Read the model definition and answer for the solid it produces. Units are mm, in the model's axes. A direction names the side the tool comes from. Round coordinates to 2 decimals unless told otherwise and drop trailing zeros. Write each loop counter-clockwise with the first axis right and the second up, starting at its lowest first coordinate (ties: lowest second). Pieces come first, ordered by that corner, then holes. Notation, with made-up numbers: (9, -32) -> (21, -32) arc R31 cw to (21, -3) -> close; hole circle Ø5 at (12.5, 20). An arc over 180 degrees is marked (long way). Return JSON: item names as keys, results as strings.
Autodesk Inventor part; units mm, degrees
ref_plane "YZ Plane" through (0, 0, 0) normal (1, 0, 0) x (0, 1, 0)
ref_plane "XZ Plane" through (0, 0, 0) normal (0, 1, 0) x (-1, 0, 0)
ref_plane "XY Plane" through (0, 0, 0) normal (0, 0, 1) x (1, 0, 0)
sketch "Эскиз1" plane through (0, 0, 0) normal (0, 1, 0) x (-1, 0, 0)
  line L0 (0, 0) -> (-2.8, 0)
  line L1 (0, 0) -> (0, -6)
  line L2 (0, -6) -> (-1.3212, -6)
  line L3 (-1.45, -5.8712) -> (-1.45, -1.65)
  line L4 (-2.8, -0.3) -> (-1.45, -1.65)
  line L5 (-2.8, 0) -> (-2.8, -0.3)
  line L6 (-1.45, -5.8712) -> (-1.3212, -6)
revolve "Вращение1" add sketch "Эскиз1" angle 360 about axis through (0, 0, 0) along (0, 0, -1)
sketch "Эскиз2" plane through (0, 0, 0) normal (0, 0, 1) x (1, 0, 0)
  line L0 (-1.3212, -0.4705) -> (-1.3212, 0.4705)
  line L1 (1.3212, 0.4705) -> (1.3212, -0.4705)
  circle A0 centre (0, 0) radius 1.45
  line L2 (0.4865, -1.366) -> (-0.4865, -1.366)
  line L3 (-0.4865, 1.366) -> (0.4865, 1.366)
  line L4 (1.3212, -0.4705) -> (0.4865, -0.4705)
  line L5 (-0.4865, -0.4705) -> (-1.3212, -0.4705)
  line L6 (-0.4865, -1.366) -> (-0.4865, -0.4705)
  line L7 (-0.4865, 0.4705) -> (-0.4865, 1.366)
  line L8 (-1.3212, 0.4705) -> (-0.4865, 0.4705)
  line L9 (0.4865, 0.4705) -> (1.3212, 0.4705)
  line L10 (0.4865, 1.366) -> (0.4865, 0.4705)
  line L11 (0.4865, -0.4705) -> (0.4865, -1.366)
extrude "Выдавливание1" cut sketch "Эскиз2" against normal blind 1 contours L0 L8 L7 L3 L10 L9 L1 L4 L11 L2 L6 L5
thread "Резьба1"
properties part number "Винт М3х6 пот"
Item 1: Section C-C (x = 0) is taken. Give the vertices of the cut face in (y, z), then the cut area to 3 significant figures.
Worked answers:
{"outline": "(-2.8, -0.3) -> (-1.45, -1.65) -> (-1.45, -5.87) -> (-1.32, -6) -> (1.32, -6) -> (1.45, -5.87) -> (1.45, -1.65) -> (2.8, -0.3) -> (2.8, 0) -> (1.37, 0) -> (1.37, -1) -> (-1.37, -1) -> (-1.37, 0) -> (-2.8, 0) -> close", "area": "17.3 mm2"}
Item 2: Section D-D (z = -2.75) is taken. Give the vertices of the cut face in (x, y), then the cut area to 3 significant figures.
Worked answers:
{"outline": "circle Ø2.9 at (0, 0)", "area": "6.61 mm2"}
Item 3: Straight lines are drawn through the part: L1, parallel to X at y = -0.05, z = -0.25; L2, parallel to Y at x = 0.05, z = -1.7; L3, parallel to Z at x = -0.1, y = 2.1. For each, find the intervals that lie inside material, in ascending order. Write a range as [from, to].
Worked answers:
{"L1": "x = [-2.8, -1.32], [1.32, 2.8]", "L2": "y = [-1.45, 1.45]", "L3": "z = [-1, 0]"}
Item 4: A tool of negligible diameter and unlimited length cuts with its end or side. For faces 4 (the flat face through (-0.9, -0.47, -0.5)), 5 (the flat face through (1, 1, 0)), from which of +Z, -Z, +X, -X, +Y, -Y can it reach the whole face along a straight path? Write none if from no direction.
Worked answers:
{"face 4": "+Z", "face 5": "+Z, +X, -X, +Y, -Y"}
Item 5: Section A-A (z = -0.5) is taken. Give the vertices of the cut face in (x, y), then the cut area to 3 significant figures.
Worked answers:
{"outline": "circle Ø5.2 at (0, 0); hole (-1.32, -0.47) -> (-0.49, -0.47) -> (-0.49, -1.37) -> (0.49, -1.37) -> (0.49, -0.47) -> (1.32, -0.47) -> (1.32, 0.47) -> (0.49, 0.47) -> (0.49, 1.37) -> (-0.49, 1.37) -> (-0.49, 0.47) -> (-1.32, 0.47) -> close", "area": "17.0 mm2"}
Item 6: For a pull along X with two mould halves and no side action, classify faces 1 (the cylindrical face through (-1.45, 0.06, -3.73)), 2 (the flat face through (0, 0, -6)), 3 (the flat face through (0.486, 0.9, -0.5)) as released by +X, released by -X, zero draft, split by the parting line, or undercut.
Worked answers:
{"face 1": "split by the parting line", "face 2": "zero draft", "face 3": "undercut"}
Item 7: Section B-B (y = 0) is taken. Give the vertices of the cut face in (x, z).
Worked answers:
{"outline": "(-2.8, -0.3) -> (-1.45, -1.65) -> (-1.45, -5.87) -> (-1.32, -6) -> (1.32, -6) -> (1.45, -5.87) -> (1.45, -1.65) -> (2.8, -0.3) -> (2.8, 0) -> (1.32, 0) -> (1.32, -1) -> (-1.32, -1) -> (-1.32, 0) -> (-2.8, 0) -> close"}
Item 8: Flat-ended cylindrical pins translate along their axes: pin 1 (0.8 mm diameter, centred on y = 0, z = -0.5, fed in from -X); pin 2 (1 mm diameter, centred on y = -1, z = -0.5, fed in from -X); pin 3 (1.5 mm diameter, centred on x = 0, z = -3.5, fed in from +Y); pin 4 (3 mm diameter, centred on y = 1.5, z = -5.5, fed in from +X). Find the tip coordinate at first contact, or state that the pin passes through.
Worked answers:
{"pin 1": "stops at x = -2.8", "pin 2": "stops at x = -2.75", "pin 3": "stops at y = 1.45", "pin 4": "stops at x = 1.45"}
